Can you work these out from the model? Positions are in its coordinate system, mm. Face numbers are marked on the shaded views. A direction names the side the tool comes from. Give positions to 0.01 mm unless a question says otherwise; leave off trailing zeros. Order: outer loops, then holes, each group sorted by start corner. A loop starts at its lowest first (then second) coordinate and runs counter-clockwise, first axis right, second up. Notation, with made-up numbers: M 24,-31 L 57,-31 A25 ccw 57,-11 Z; hole C 0.25,20 d6. An arc over 180 degrees is marked long. Answer as a JSON object with one key per item and string values.
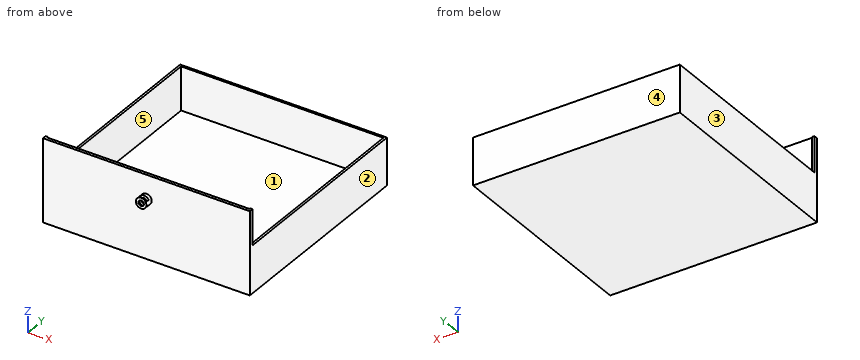
```python
from build123d import *

# Parameters (mm, degrees)
F0_W      = 125.476
F0_H      = 50.292
F1_DEPTH  = 125.476
F2_W      = 122.7189972997
F2_H      = 122.4945134018
F3_DEPTH  = 48.006
F5_R      = 3.2177672419
F5_R_2    = 1.6781805888
F6_DEPTH  = 4.826
F7_W      = 80.5568695068
F7_H      = 21.6923308617
F8_DEPTH  = 125.477
F9_W      = 42.4876958132
F9_H      = 25.0391000882
F10_DEPTH = 125.477
F11_W     = 5.6567939464
F11_H     = 2.2512227297
F12_DEPTH = 48.007


# Not quite as in the source:
# - a feature names something its author has since deleted; it is built from what else it names


with BuildPart() as f1:
    # F0 (on Front) → F1 (new body)
    with BuildSketch(Plane.XZ):
        Rectangle(F0_W, F0_H)
    extrude(amount=F1_DEPTH)

    # F2 (on face) → F3 (cut)
    with BuildSketch(Plane.XY.offset(25.146)):
        with Locations((7.4506e-06, -62.4770697905)):
            Rectangle(F2_W, F2_H)
    extrude(amount=-F3_DEPTH, mode=Mode.SUBTRACT)

    # F5 (on face) → F6 (join)
    with BuildSketch(Plane.XZ.offset(125.476)):
        with Locations((0, 10.6488130987)):
            Circle(F5_R)
        with Locations((0, 10.6488130987)):
            Circle(F5_R_2, mode=Mode.SUBTRACT)
    extrude(amount=F6_DEPTH)

    # F7 (on face) → F8 (cut, through all)
    with BuildSketch(Plane.YZ.offset(62.738)):
        with Locations((-40.2784347534, 14.2998345691)):
            Rectangle(F7_W, F7_H)
    extrude(amount=-F8_DEPTH, mode=Mode.SUBTRACT)

    # F9 (on face) → F10 (cut, through all)
    with BuildSketch(Plane.YZ.offset(62.738)):
        with Locations((-101.8007174134, 15.9732191823)):
            Rectangle(F9_W, F9_H)
    extrude(amount=-F10_DEPTH, mode=Mode.SUBTRACT)

    # F11 (on face) → F12 (cut, through all)
    with BuildSketch(Plane.XY.offset(-22.86)):
        with Locations((-0.0043596374, -128.7486031651)):
            Rectangle(F11_W, F11_H)
    extrude(amount=F12_DEPTH, mode=Mode.SUBTRACT)


solid = f1.part
```
1) For the marked faces 4 and 5, which set-ups out of +Z, -Z, +X, -X, +Y, -Y let a thin tool reach every point of the face, with its end or its side?
Results found:
{"face 4": "+Z, -Z, +X, -X, +Y", "face 5": "+Z"}
2) I'm going to push flat-ended pins straight in: pin 1 Ø4 at (x, z) = (22, 12) entering from +Y; pin 2 Ø8 at (x, y) = (16, -66) entering from +Z; pin 3 Ø1.5 at (x, z) = (62, 15.5) entering from +Y. Where does each tip first touch, or does it pass through?
Results found:
{"pin 1": "stops at y = -123.72", "pin 2": "stops at z = -22.86", "pin 3": "stops at y = -123.04"}
3) I want a section at A-A on x = 0. Write out the boundary of the cut face in (y, z), and give its area (3 significant figures).
Results found:
{"outline": "M -130.3,7.43 L -129.87,7.43 L -129.87,8.97 L -130.3,8.97 Z; M -130.3,12.33 L -129.87,12.33 L -129.87,13.87 L -130.3,13.87 Z; M -127.62,7.43 L -125.48,7.43 L -125.48,-25.15 L 0,-25.15 L 0,3.45 L -1.23,3.45 L -1.23,-22.86 L -123.72,-22.86 L -123.72,25.15 L -125.48,25.15 L -125.48,13.87 L -127.62,13.87 L -127.62,12.33 L -125.48,12.33 L -125.48,8.97 L -127.62,8.97 Z", "area": "411 mm²"}
4) Thinking about a two-plate mould opening in X: for the marked faces 1, 2 and 3, which applies, pulls with the +X half, pulls with the -X half, needs draft (parallel to the pull), parting line crosses it, or undercut?
Results found:
{"face 1": "undercut", "face 2": "pulls with the +X half", "face 3": "pulls with the -X half"}
5) I want a section at D-D on x = -42.5. Write out the boundary of the cut face in (y, z).
Results found:
{"outline": "M -125.48,-25.15 L 0,-25.15 L 0,3.45 L -1.23,3.45 L -1.23,-22.86 L -123.72,-22.86 L -123.72,25.15 L -125.48,25.15 Z"}
6) I want a section at B-B on z = -15. Write out the boundary of the cut face in (x, y), and give its area (3 significant figures).
Results found:
{"outline": "M -62.74,-125.48 L 62.74,-125.48 L 62.74,0 L -62.74,0 Z; hole M -61.36,-123.72 L 61.36,-123.72 L 61.36,-1.23 L -61.36,-1.23 Z", "area": "712 mm²"}
7) I need wall thicknesses on L1, parallel to X at y = -97.5, z = -8; L2, parallel to Y at x = 22, z = -13; L3, parallel to Z at x = 0, y = -126.25. Which ranges of each line are inside material? Lowest first, please.
Results found:
{"L1": "x = -62.74 to -61.36, 61.36 to 62.74", "L2": "y = -125.48 to -123.72, -1.23 to 0", "L3": "z = 7.43 to 8.97, 12.33 to 13.87"}
8) I want a section at C-C on y = -22. Write out the boundary of the cut face in (x, z), and give its area (3 significant figures).
Results found:
{"outline": "M -62.74,-25.15 L 62.74,-25.15 L 62.74,3.45 L 61.36,3.45 L 61.36,-22.86 L -61.36,-22.86 L -61.36,3.45 L -62.74,3.45 Z", "area": "359 mm²"}
